from build123d import *

# Parameters (mm, degrees)
SKETCH1_R            = 45
SKETCH1_R_2          = 41
BOSS_EXTRUDE1_DEPTH  = 3
SKETCH2_R            = 1.459793725
BOSS_EXTRUDE2_DEPTH  = 3
CUT_EXTRUDE1_DEPTH   = 3
FILLET1_R            = 10
FILLET1_OF_MIRROR1_R = 10


with BuildPart() as part:
    # Sketch1 → Boss-Extrude1 (new body)
    with BuildSketch(Plane.XY):
        Circle(SKETCH1_R)
        Circle(SKETCH1_R_2, mode=Mode.SUBTRACT)
    extrude(amount=BOSS_EXTRUDE1_DEPTH)

    # Sketch2 → Boss-Extrude2 (add)
    with BuildSketch(Plane.XY.offset(3)):
        with BuildLine():
            Line((-15.668886268, 42.183954332), (-19.883661907, 35.855822249))
            add(Edge.make_bspline(
                [(-12.086416771, 32.285039051), (-12.597852714, 39.589288788), (-19.883661907, 35.855822249)],
                knots=[0, 0, 0, 1, 1, 1], degree=2))
            ThreePointArc((-12.086416771, 32.285039051), (-8.086416771, 28.285039051), (-4.086416771, 32.285039051))
            add(Edge.make_bspline(
                [(-4.086416771, 32.285039051), (-3.775529113, 34.928467106), (-6.013218517, 41.206349148), (-12.686993609, 42.383352938), (-15.668886268, 42.183954332)],
                knots=[0, 0, 0, 0, 0.461232636, 1, 1, 1, 1], degree=3))
        make_face()
        with Locations((-8.086416771, 32.285039051)):
            Circle(SKETCH2_R, mode=Mode.SUBTRACT)
    boss_extrude2 = extrude(amount=-BOSS_EXTRUDE2_DEPTH)

    # Sketch3 → Cut-Extrude1 (cut)
    with BuildSketch(Plane.XY.offset(3)):
        Polygon((0, 45), (0, 37.437139849), (-7.602836832, 40.288917485), (-11.716734304, 43.447878398), (-6.589372727, 48.458841459), align=None)
    cut_extrude1 = extrude(amount=-CUT_EXTRUDE1_DEPTH, mode=Mode.SUBTRACT)

    # Fillet1
    # the kernel refuses this fillet: 10 mm, written as the material it takes off along each edge
    with BuildSketch(Plane(origin=(-11.716734304, 43.447878398, 18.140851252), x_dir=(-0.9457987516283185, -0.32475332395268036, 0), z_dir=(0, 0, -1))) as fillet1_piece_1:
        with BuildLine():
            CenterArc((5.383413779, -9.977332791), FILLET1_R, 86.141498066, 59.431279914)
            Line((-2.865036036, -4.323743166), (-3.030005033, -4.210671374))
            ThreePointArc((-3.030005033, -4.210671374), (-1.599238142, -2.051398055), (-0.166720124, 0.110473528))
            Line((-0.166720124, 0.110473528), (-0.013458534, 0.199546656))
            ThreePointArc((-0.013458534, 0.199546656), (3.02817025, 0.30200244), (6.069799035, 0.199546656))
            Line((6.069799035, 0.199546656), (6.056340501, 0))
        make_face()
    extrude(amount=33.281702504, mode=Mode.SUBTRACT)

    # Mirror1: Boss-Extrude2, Cut-Extrude1 across plane
    add(boss_extrude2.mirror(Plane(origin=(0, 0, 0), x_dir=(0, 0, 1), z_dir=(1, 0, 0))))
    add(cut_extrude1.mirror(Plane(origin=(0, 0, 0), x_dir=(0, 0, 1), z_dir=(1, 0, 0))), mode=Mode.SUBTRACT)

    # Fillet1 of Mirror1
    # the kernel refuses this fillet: 10 mm, written as the material it takes off along each edge
    with BuildSketch(Plane(origin=(11.716734304, 43.447878398, 18.140851252), x_dir=(0.9457987516283181, -0.324753323952681, 0), z_dir=(0, 0, -1))) as fillet1_of_mirror1_piece_1:
        with BuildLine():
            CenterArc((5.383413779, 9.977332791), FILLET1_OF_MIRROR1_R, 214.42722202, 59.431279914)
            Line((-2.865036036, 4.323743166), (-3.030005033, 4.210671374))
            ThreePointArc((-3.030005033, 4.210671374), (-1.599238142, 2.051398055), (-0.166720124, -0.110473528))
            Line((-0.166720124, -0.110473528), (-0.013458534, -0.199546656))
            ThreePointArc((-0.013458534, -0.199546656), (3.02817025, -0.30200244), (6.069799035, -0.199546656))
            Line((6.069799035, -0.199546656), (6.056340501, 0))
        make_face()
    extrude(amount=33.281702504, mode=Mode.SUBTRACT)


solid = part.part
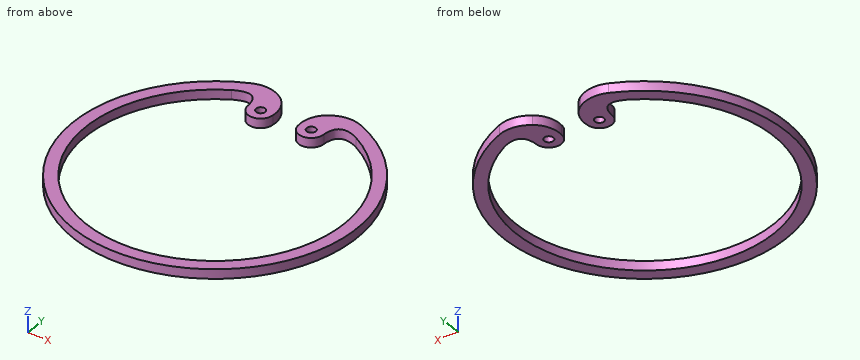
For this review, take the finished solid that the model builds, in its own axes (mm). Coordinates: 2 decimals unless noted, no trailing zeros. Order: outer loops, then holes, each group sorted by start corner. A loop starts at its lowest first (then second) coordinate and runs counter-clockwise, first axis right, second up. Notation, with made-up numbers: (-16.75, 10.5) - (11.25, 10.5) arc R23 cw to (11.25, 18.5) - close; hole circle Ø8 at (-9.75, 31.5). An arc over 180 degrees is marked (long way). Use one line per item in the form item = value.
Q1. Consider section B-B (x = 35). Give the boundary of the cut face in (y, z), then the cut area to 3 significant figures.
Checked values:
outline = (-28.28, 0) - (-21.35, 0) - (-21.35, 3) - (-28.28, 3) - close; (21.35, 0) - (28.28, 0) - (28.28, 3) - (21.35, 3) - close
area = 41.6 mm2
Q2. Consider section C-C (z = 1.4). Give the number of separate pieces and of enclosed holes in the cut face, then the cut area to 3 significant figures.
Checked values:
separate_pieces = 1
enclosed_holes = 2
area = 1,160 mm2
Q3. For P1, Ø1, axis at x = -7.5, z = 2, coming from the +Y side; P2, Ø1.5, axis at y = -5, z = 0.5, coming from the +X side, all flat-tipped, find the tip position at first contact; note any pin that passes through.
Checked values:
P1 = 40.57
P2 = 44.8
Q4. For probe 1 along X at (y, z) = (0, 1.65); probe 2 along Y at (x, z) = (-7, 1.9); probe 3 along X at (y, z) = (-29, 1.55), list the stretches that pass through material, from the lowest coordinate up. Write a range as from..to.
Checked values:
probe_1 = -45..-41, 41..45
probe_2 = -44.45..-40.4, 28.44..31.31, 33.26..39.83
probe_3 = -34.41..-28.98, 28.98..34.41
Q5. Consider section A-A (y = 0). Give the boundary of the cut face in (x, z).
Checked values:
outline = (-45, 0) - (-41, 0) - (-41, 3) - (-45, 3) - close; (41, 0) - (45, 0) - (45, 3) - (41, 3) - close
Q6. Consider section D-D (x = 0). Give the boundary of the cut face in (y, z).
Checked values:
outline = (-45, 0) - (-41, 0) - (-41, 3) - (-45, 3) - close
